Could you check a few things on this model? Use its own coordinates, in mm. Face numbers are marked on the shaded views. A direction names the side the tool comes from. Round coordinates to 2 decimals unless told otherwise and drop trailing zeros. Write each loop counter-clockwise with the first axis right and the second up, starting at its lowest first coordinate (ties: lowest second). Pieces come first, ordered by that corner, then holes. Notation, with made-up numbers: (38, -2) -> (54, -2) arc R20 ccw to (54, 17) -> close; hole circle Ø5 at (69, -4). An arc over 180 degrees is marked (long way). Answer in a Markdown table with one row per item. Add a question column.
```python
from build123d import *

# Parameters (mm, degrees)
F1_DEPTH = 17.78
F2_DEPTH = 12.7
F3_DEPTH = 127
F4_DEPTH = 50.8


with BuildPart() as f1:
    # F0 (on Front) → F1 (new body)
    with BuildSketch(Plane.XZ):
        Polygon((-26.9799930214, -30.0789192878), (-1.3335170985, -40.384194199), (24.9369262952, -31.7932558242), (39.5391047323, -8.3258997066), (35.640496637, 19.0372374158), (15.0653040652, 37.492639576), (-0.0947250793, 37.9932353779), (-0.2021778175, 34.7391396875), (-10.0282026626, 27.4203366243), (-12.1426928308, 27.9769725351), (-11.8020968639, 20.0453100056), (-27.8368135787, 6.0916620046), (-37.1591211673, 7.8023393187), (-40.0022303604, -5.6993837518), align=None)
    extrude(amount=F1_DEPTH)

    # F0 (on Front) → F2 (join)
    with BuildSketch(Plane.XZ):
        Polygon((-48.7436972284, 9.9281511173), (-37.1591211673, 7.8023393187), (-34.3069795385, 21.3469567832), (-22.0594268614, 30.9532808442), (-26.8255087596, 41.7476859043), (-23.1050903168, 48.862511609), (-29.8858768711, 53.8094276768), (-50.3869184057, 48.1948280781), (-58.7794380023, 28.6658227916), align=None)
        Polygon((-34.3069795385, 21.3469567832), (-37.1591211673, 7.8023393187), (-27.8368135787, 6.0916620046), (-11.8020968639, 20.0453100056), (-12.1426928308, 27.9769725351), (-21.8766995951, 30.539433124), (-22.0594268614, 30.9532808442), align=None)
    extrude(amount=F2_DEPTH)

    # F0 (on Front) → F3 (join)
    with BuildSketch(Plane.XZ):
        Polygon((-12.5591117109, 38.4048189943), (-0.0947250793, 37.9932353779), (0.2021778175, 46.9846343306), (-9.1196237983, 54.9357133249), (-21.1480759179, 52.6050520151), (-23.1050903168, 48.862511609), (-12.7140158191, 41.2817135729), (-12.589456174, 38.3810184234), align=None)
        Polygon((-0.2021778175, 34.7391396875), (-0.0947250793, 37.9932353779), (-12.5591117109, 38.4048189943), (-12.589456174, 38.3810184234), (-12.1426928308, 27.9769725351), (-10.0282026626, 27.4203366243), align=None)
        Polygon((-26.8255087596, 41.7476859043), (-22.0594268614, 30.9532808442), (-12.589456174, 38.3810184234), (-12.7140158191, 41.2817135729), (-23.1050903168, 48.862511609), align=None)
        Polygon((-12.589456174, 38.3810184234), (-22.0594268614, 30.9532808442), (-21.8766995951, 30.539433124), (-12.1426928308, 27.9769725351), align=None)
    extrude(amount=F3_DEPTH)

    # F0 (on Front) → F4 (cut)
    with BuildSketch(Plane.XZ):
        Polygon((-26.8255087596, 41.7476859043), (-22.0594268614, 30.9532808442), (-12.589456174, 38.3810184234), (-12.7140158191, 41.2817135729), (-23.1050903168, 48.862511609), align=None)
        Polygon((-12.5591117109, 38.4048189943), (-0.0947250793, 37.9932353779), (0.2021778175, 46.9846343306), (-9.1196237983, 54.9357133249), (-21.1480759179, 52.6050520151), (-23.1050903168, 48.862511609), (-12.7140158191, 41.2817135729), (-12.589456174, 38.3810184234), align=None)
        Polygon((-0.2021778175, 34.7391396875), (-0.0947250793, 37.9932353779), (-12.5591117109, 38.4048189943), (-12.589456174, 38.3810184234), (-12.1426928308, 27.9769725351), (-10.0282026626, 27.4203366243), align=None)
        Polygon((-12.589456174, 38.3810184234), (-22.0594268614, 30.9532808442), (-21.8766995951, 30.539433124), (-12.1426928308, 27.9769725351), align=None)
    extrude(amount=-F4_DEPTH, mode=Mode.SUBTRACT)


solid = f1.part
```
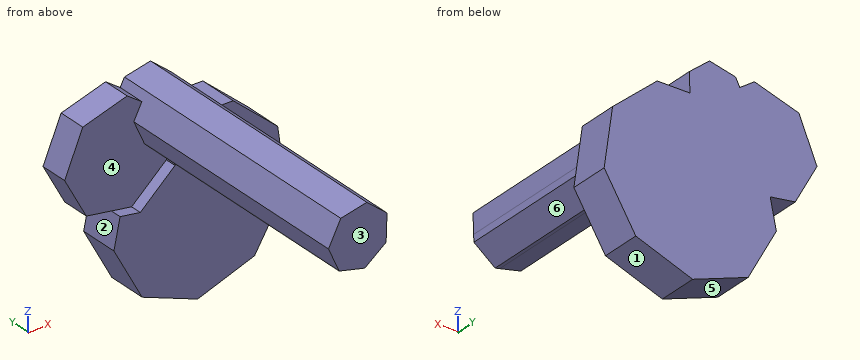
(1) Suppose I cut it at D-D, the plane z = -24.5. Please give me the cut outline in (x, y).
(2) I need wall thicknesses on L1, parallel to Y at x = -16, z = 13.5; L2, parallel to Z at x = -15.5, y = -17.5; L3, parallel to Y at x = -37, z = 23.5. Which ranges of each line are inside material? Lowest first, please.
(3) Suppose I cut it at C-C, the plane z = 17. Please give me the cut outline in (x, y).
(4) For P1, Ø6, axis at x = 5, y = -66, coming from the -Z side; P2, Ø23.5, axis at x = 3, z = -7, coming from the -Y side; P3, Ø6, axis at x = -37, z = 43, coming from the -Y side; P4, Ø1, axis at x = -17, y = -93.5, coming from the -Z side, each with a flat end and sliding along its axis, tell me the tip position at first contact or that it passes through.
(5) If we mould it in two halves opening along Z, with no side actions, what happens to the marked faces 1, 2, 3 and 4? For each: pulls with the +Z half, pulls with the -Z half, needs draft (parallel to the pull), parting line crosses it, or undercut.
(6) Suppose I cut it at B-B, the plane x = -34.5. Please give me the cut outline in (y, z).
(7) Suppose I cut it at A-A, the plane y = -78.5. Please give me the cut outline in (x, z), then the cut area to 3 significant figures.
(8) On a 3-axis mill with a long thin cutter (end or side, diameter ignored), from which of +Z, -Z, +X, -X, +Y, -Y can I reach the whole of each face in a straight line? I mean the marked faces 5 and 6. Say none if no direction works.
Response:
| question | item | result |
|---|---|---|
| 1 | outline | (-29.96, -17.78) -> (29.48, -17.78) -> (29.48, 0) -> (-29.96, 0) -> close |
| 2 | L1 | -17.78 to 0 |
| 2 | L2 | -34.69 to 16.83, 28.86 to 53.7 |
| 2 | L3 | -12.7 to 0 |
| 3 | outline | (-52.53, -12.7) -> (-15.3, -12.7) -> (-15.3, -17.78) -> (35.93, -17.78) -> (35.93, 0) -> (-52.53, 0) -> close |
| 4 | P1 | through |
| 4 | P2 | y = -17.78 |
| 4 | P3 | y = -12.7 |
| 4 | P4 | z = 29.12 |
| 5 | face 1 | pulls with the -Z half |
| 5 | face 2 | undercut |
| 5 | face 3 | needs draft |
| 5 | face 4 | undercut |
| 6 | outline | (-17.78, -16) -> (0, -16) -> (0, 52.55) -> (-12.7, 52.55) -> (-12.7, 7.31) -> (-17.78, 7.31) -> close |
| 7 | outline | (-26.83, 41.75) -> (-21.88, 30.54) -> (-10.03, 27.42) -> (-0.2, 34.74) -> (0.2, 46.98) -> (-9.12, 54.94) -> (-21.15, 52.61) -> close |
| 7 | area | 546 mm² |
| 8 | face 5 | -Z, -X, +Y, -Y |
| 8 | face 6 | -Z, +X, -Y |
